Check sheet for the modelled part. Datum: model origin and axes. Units: mm. A direction names the side the tool comes from. Coordinates: 2 decimals unless noted, no trailing zeros. Write each loop counter-clockwise with the first axis right and the second up, starting at its lowest first coordinate (ties: lowest second). Pieces come first, ordered by that corner, then holes. Notation, with made-up numbers: (80.25, 72.25) -> (96.25, 72.25) arc R22 ccw to (96.25, 91.25) -> close; hole circle Ø1 at (14.5, 54.25). An arc over 180 degrees is marked (long way). Put each result on its own line as item: value.
Autodesk Inventor part; units mm, degrees
ref_plane "YZ Plane" through (0, 0, 0) normal (1, 0, 0) x (0, 1, 0)
ref_plane "XZ Plane" through (0, 0, 0) normal (0, 1, 0) x (-1, 0, 0)
ref_plane "XY Plane" through (0, 0, 0) normal (0, 0, 1) x (1, 0, 0)
sketch "スケッチ1" plane through (0, 0, 0) normal (0, 1, 0) x (-1, 0, 0)
  line L0 (-21.25, 21.25) -> (21.25, 21.25)
  line L1 (21.25, 21.25) -> (21.25, -21.25)
  line L2 (21.25, -21.25) -> (-21.25, -21.25)
  line L3 (-21.25, -21.25) -> (-21.25, 21.25)
  line L4 (-21.25, 21.25) -> (21.25, -21.25) construction
  line L5 (21.25, 21.25) -> (-21.25, -21.25) construction
  line L6 (-21.25, 27.5) -> (-16.25, 27.5)
  line L7 (-16.25, 27.5) -> (-16.25, -27.5)
  line L8 (-16.25, -27.5) -> (-21.25, -27.5)
  line L9 (-21.25, -27.5) -> (-21.25, 27.5)
  line L10 (-21.25, 27.5) -> (-16.25, -27.5) construction
  line L11 (-16.25, 27.5) -> (-21.25, -27.5) construction
  line L12 (21.25, 21.25) -> (-16.25, 27.5)
  line L13 (-16.25, -27.5) -> (21.25, -21.25)
  point P0 (0, 0)
  point P1 (-18.75, 0)
  dimension "d0" = 42.5
  dimension "d1" = 42.5
  dimension "d12" = 6.25
  dimension "d13" = 5
extrude "プレート1" add sketch "スケッチ1" along normal blind 5
sketch "スケッチ2" plane through (0, 5, 0) normal (0, 1, 0) x (1, 0, 0)
  line L0 (15.5, -15.5) -> (-15.5, -15.5) construction
  line L1 (-15.5, -15.5) -> (-15.5, 15.5) construction
  line L2 (-15.5, 15.5) -> (15.5, 15.5) construction
  line L3 (15.5, 15.5) -> (15.5, -15.5) construction
  line L4 (15.5, -15.5) -> (-15.5, 15.5) construction
  line L5 (-15.5, -15.5) -> (15.5, 15.5) construction
  point P0 (0, 0)
  dimension "d3" = 31
  dimension "d4" = 31
hole "穴1" at (15.5, 5, 15.5) at (15.5, 5, -15.5) at (-15.5, 5, -15.5) at (-15.5, 5, 15.5) direction (0, -1, 0) diameter 3.5 depth 5 tip angle 118 counterbore diameter 6 counterbore depth 3
sketch "スケッチ3" plane through (0, 5, 0) normal (0, 1, 0) x (1, 0, 0)
  line L0 (21.25, 27.5) -> (21.25, -27.5)
  circle A0 centre (22.1, -22.5) radius 1.05
  line L1 (21.25, -27.5) -> (16.25, -27.5)
  line L2 (16.25, -27.5) -> (-21.25, -21.25)
  line L3 (-11.5, -20.8474) -> (16.25, -25.4724)
  line L4 (16.25, -25.4724) -> (16.25, -20.5518)
  line L5 (16.25, -20.5518) -> (9.2321, -16.5)
  line L6 (9.2321, -16.5) -> (-11.5, -16.5)
  line L7 (-11.5, -16.5) -> (-11.5, -20.8474)
  line L8 (-21.25, -21.25) -> (-21.25, 21.25)
  circle A1 centre (15.5, -15.5) radius 1.75
  circle A2 centre (-15.5, -15.5) radius 1.75
  point P0 (0, 0)
  dimension "d14" = 2.1
  dimension "d15" = 0.85
  dimension "d16" = 5
  dimension "d19" = 2
  dimension "d20" = 5
  dimension "d21" = 4
  dimension "d22" = 1
  dimension "d23" = 4
  dimension "d24" = 120
extrude "押し出し1" cut sketch "スケッチ3" against normal through all contours A0 L0 | L0 A0 | L7 L6 L5 L4 L3
fillet "フィレット1" radius 2 5 edges at (16.25, 2.5, 25.4724) (16.25, 2.5, 20.5518) (9.2321, 2.5, 16.5) (-11.5, 2.5, 16.5) (-11.5, 2.5, 20.8474)
sketch "スケッチ4" plane through (21.25, 0, 27.5) normal (1, 0, 0) x (0, 0, -1)
  line L0 (4.3836, 0) -> (4.3836, 5)
  line L1 (5.6164, 0) -> (4.3836, 0)
  line L2 (5.6164, 5) -> (5.6164, 0)
  line L3 (4.3836, 5) -> (5.6164, 5)
  point P0 (27.5, 0)
  point P1 (5, 2.5)
  point P2 (5, 5)
  point P3 (4.3836, 2.5)
hole "穴2" at (21.25, 2.5, 22.5) direction (-1, 0, 0) diameter 2.5 depth 8 tip angle 118
mirror "ミラー1" about plane through (0, 0, 0) normal (0, 0, 1) of "押し出し1", "フィレット1", "穴2"
sketch "スケッチ5" plane through (0, 5, 0) normal (0, 1, 0) x (1, 0, 0)
  circle A0 centre (0, 0) radius 13.5
  dimension "d33" = 27
extrude "押し出し2" cut sketch "スケッチ5" against normal through all
fillet "フィレット2" radius 2 6 edges at (-21.25, 2.5, 21.25) (-21.25, 2.5, -21.25) (16.25, 2.5, -27.5) (21.25, 2.5, -27.5) (21.25, 2.5, 27.5) (16.25, 2.5, 27.5)
sketch "スケッチ6" plane through (0, 5, 0) normal (0, 1, 0) x (1, 0, 0)
  line L0 (-21.25, -19.5557) -> (-21.25, 19.5557)
  circle A0 centre (-22.1, 0) radius 1.05
  point P0 (0, 0)
  dimension "d37" = 2.1
  dimension "d38" = 0.85
extrude "押し出し3" cut sketch "スケッチ6" against normal through all
sketch "スケッチ7" plane through (0, 5, 0) normal (0, 1, 0) x (1, 0, 0)
  line L0 (-16.7, -7.5) -> (-16.7, 7.5) construction
  line L1 (-15.65, -7.5) -> (-15.65, 7.5)
  line L2 (-17.75, 7.5) -> (-17.75, -7.5)
  arc A0 (-17.75, -7.5) -> (-15.65, -7.5) centre (-16.7, -7.5) ccw
  arc A1 (-15.65, 7.5) -> (-17.75, 7.5) centre (-16.7, 7.5) ccw
  line L3 (-21.25, 0.6164) -> (-21.25, 19.5557)
  point P0 (0, 0)
  point P1 (-16.7, 0)
  dimension "d41" = 3.5
  dimension "d42" = 2.1
  dimension "d43" = 15
extrude "押し出し4" cut sketch "スケッチ7" against normal through all
sketch "スケッチ8" plane through (-21.25, 0, 19.5557) normal (-1, 0, 0) x (0, 0, 1)
  line L0 (-20.1722, 0) -> (-20.1722, 5)
  line L1 (-18.9393, 0) -> (-20.1722, 0)
  line L2 (-18.9393, 5) -> (-18.9393, 0)
  line L3 (-20.1722, 5) -> (-18.9393, 5)
  point P0 (-19.5557, 0)
  point P1 (-19.5557, 2.5)
  point P2 (-19.5557, 0)
  point P3 (-18.9393, 2.5)
hole "穴3" at (-21.25, 2.5, 0) direction (1, 0, 0) diameter 2.5 depth 4 tip angle 118
equation "\"d10\" = Thickness"
equation "\"d23\" = d21"
equation "\"d2\" = Thickness"
equation "\"BendRadius\" = Thickness"
equation "\"BendReliefWidth\" = Thickness"
equation "\"BendReliefDepth\" = 0.5 * Thickness"
equation "\"TransitionRadius\" = BendRadius"
equation "\"JacobiRadiusSize\" = BendRadius"
equation "\"GapSize\" = Thickness"
properties part number "T5.0_stepper-fix"
Q1. Cross-section at B-B (x = -6). Record the cut outline in (y, z).
Recorded:
outline: (0, -23.79) -> (5, -23.79) -> (5, -21.76) -> (0, -21.76) -> close; (0, -16.5) -> (5, -16.5) -> (5, -12.09) -> (0, -12.09) -> close; (0, 12.09) -> (5, 12.09) -> (5, 16.5) -> (0, 16.5) -> close; (0, 21.76) -> (5, 21.76) -> (5, 23.79) -> (0, 23.79) -> close
Q2. Depth check by flat-ended pin: P1, Ø1.8, axis at x = -14, z = 16, coming from the +Y side. Enter the tip coordinate at first touch or a pass-through.
Recorded:
P1: stops at y = 2
Q3. Cross-section at C-C (z = 15.5). Record the cut outline in (x, y).
Recorded:
outline: (-21.25, 0) -> (-17.25, 0) -> (-17.25, 2) -> (-18.5, 2) -> (-18.5, 5) -> (-21.25, 5) -> close; (-13.75, 0) -> (13.75, 0) -> (13.75, 2) -> (12.5, 2) -> (12.5, 5) -> (-12.5, 5) -> (-12.5, 2) -> (-13.75, 2) -> close; (17.25, 0) -> (21.25, 0) -> (21.25, 5) -> (18.5, 5) -> (18.5, 2) -> (17.25, 2) -> close
Q4. Material ranges on line 1 along X through (y, z) = (3.9, 0); line 2 along X through (y, z) = (0.55, -15.5); line 3 along Z through (x, y) = (-14.5, 3.75) (3 decimals), recorded low to high.
Recorded:
line 1: x = -21.05 to -17.75, -15.65 to -13.5, 13.5 to 21.25
line 2: x = -21.25 to -17.25, -13.75 to 13.75, 17.25 to 21.25
line 3: z = -22.375 to -18.328, -12.672 to 12.672, 18.328 to 22.375
Q5. Cross-section at D-D (z = -22.5). Record the cut outline in (x, y).
Recorded:
outline: (-13.75, 0) -> (-1.58, 0) -> (-1.58, 5) -> (-13.75, 5) -> close; (16.25, 0) -> (21.05, 0) -> (21.05, 1.25) -> (16.25, 1.25) -> close; (16.25, 3.75) -> (21.05, 3.75) -> (21.05, 5) -> (16.25, 5) -> close
Q6. Cross-section at A-A (z = 0). Record the cut outline in (x, y), plus the area to 4 significant figures.
Recorded:
outline: (-21.05, 0) -> (-17.75, 0) -> (-17.75, 1.25) -> (-21.05, 1.25) -> close; (-21.05, 3.75) -> (-17.75, 3.75) -> (-17.75, 5) -> (-21.05, 5) -> close; (-15.65, 0) -> (-13.5, 0) -> (-13.5, 5) -> (-15.65, 5) -> close; (13.5, 0) -> (21.25, 0) -> (21.25, 5) -> (13.5, 5) -> close
area: 57.75 mm2
Q7. Mould release check, pull along X, two halves, no side actions. Record for faces 5 (the cylindrical face through (-16.68, 2.54, -8.55)), 6 (the flat face through (5, 5, 13)), 7 (the flat face through (-21.25, 2, -10)): released by +X, released by -X, zero draft, split by the parting line, or undercut.
Recorded:
face 5: undercut
face 6: zero draft
face 7: released by -X
Q8. Tool access check on faces 1 (the cylindrical face through (15.524, 2.465, -24.653)), 2 (the flat face through (-2, 2.46, 24.46)), 3 (the flat face through (-14, 2, -14)), 4 (the cylindrical face through (18.662, 2.021, -21.345)). Record the directions out of +Z, -Z, +X, -X, +Y, -Y that give a thin tool (end or side, any length) a straight path to the whole face; none if there is none.
Recorded:
face 1: +Y, -Y
face 2: +Z, -X, +Y, -Y
face 3: +Y
face 4: +X
